Work out the finished part from the listing and answer in its coordinate system (mm). Round coordinates to 2 decimals unless told otherwise and drop trailing zeros. Loops run counter-clockwise (first coordinate to the right, second up) from the corner with the lowest first, then second, coordinate; pieces in that order, holes last. Notation, with made-up numbers: (-5, 84) -> (24, 84) arc R8 cw to (24, 98) -> close; hole circle Ø2 at (-40, 66). An arc over 180 degrees is marked (long way). Use one line per item in the form item = value.
```python
from build123d import *

# Parameters (mm, degrees)
F0_W     = 8.5598
F0_H     = 6.2738
F0_W_2   = 4.1402
F1_DEPTH = 1.5875
F2_D     = 3.2512


with BuildPart() as f1:
    # F0 (on Front) → F1 (new body)
    with BuildSketch(Plane.XZ):
        Polygon((0, 12.7), (-12.7, 12.7), (-12.7, -12.7), (0, -12.7), (0, -6.4262), align=None)
        Polygon((12.7, 12.7), (0, 12.7), (0, -6.4262), (8.5598, -6.4262), (12.7, -6.4262), align=None)
        with Locations((4.2799, -9.5631)):
            Rectangle(F0_W, F0_H)
        with Locations((10.6299, -9.5631)):
            Rectangle(F0_W_2, F0_H)
    extrude(amount=F1_DEPTH)

    # F2 (through all)
    with Locations(Plane(origin=(0, 0, 0), x_dir=(1, 0, 0), z_dir=(0, 1, 0))):
        with Locations((8.5598, -8.382), (-8.5852, 6.4262)):
            Hole(F2_D / 2)


solid = f1.part
```
(1) Consider L1, parallel to X at y = -1.5, z = -6.5; L2, parallel to Z at x = 8.75, y = -0.65; L3, parallel to Z at x = -9.5, y = -0.6. Determine where each line is inside the solid, lowest interval first.
Completed:
L1 = -12.7 to -10.21, -6.96 to 12.7
L2 = -12.7 to 6.77, 10 to 12.7
L3 = -12.7 to -7.77, -5.08 to 12.7
(2) Find section B-B, the plane x = -7.75. Write down the section's boundary in (y, z).
Completed:
outline = (-1.59, -12.7) -> (0, -12.7) -> (0, -7.82) -> (-1.59, -7.82) -> close; (-1.59, -5.03) -> (0, -5.03) -> (0, 12.7) -> (-1.59, 12.7) -> close
(3) Find section C-C, the plane y = -1.1. Write down the section's boundary in (x, z), then the cut area to 3 significant figures.
Completed:
outline = (-12.7, -12.7) -> (12.7, -12.7) -> (12.7, 12.7) -> (-12.7, 12.7) -> close; hole circle Ø3.25 at (-8.59, -6.43); hole circle Ø3.25 at (8.56, 8.38)
area = 629 mm2
(4) Find section A-A, the plane x = 8.5. Write down the section's boundary in (y, z), then the cut area to 3 significant figures.
Completed:
outline = (-1.59, -12.7) -> (0, -12.7) -> (0, 6.76) -> (-1.59, 6.76) -> close; (-1.59, 10.01) -> (0, 10.01) -> (0, 12.7) -> (-1.59, 12.7) -> close
area = 35.2 mm2
(5) For a pull along X with two mould halves and no side action, classify faces 1 (the cylindrical face through (8.91, -0.8, 9.97)), 2 (the flat face through (0, -1, -12.7)), 3 (the cylindrical face through (-10.087, -0.805, -5.804)), 4 (the flat face through (-12.7, -1, 0)) as +X half, -X half, draft (parallel to the pull), parting line (faces both ways), or undercut.
Completed:
face_1 = undercut
face_2 = draft
face_3 = undercut
face_4 = -X half
